The model under review builds one solid part; all positions refer to its coordinate system, in mm. Round coordinates to 2 decimals unless told otherwise and drop trailing zeros. Write each loop counter-clockwise with the first axis right and the second up, starting at its lowest first coordinate (ties: lowest second). Pieces come first, ordered by that corner, then holes. Notation, with made-up numbers: (56.25, 78) - (92.25, 78) arc R24 cw to (92.25, 96) - close; hole circle Ø4 at (-30.5, 8). An arc over 180 degrees is marked (long way). Return JSON: item names as keys, results as strings.
from build123d import *

# Parameters (mm, degrees)
F0_W     = 812.8
F0_H     = 304.8
F0_R     = 2.6924
F0_R_2   = 45.7835
F1_DEPTH = 3.81


with BuildPart() as f1:
    # F0 (on Top) → F1 (new body)
    with BuildSketch(Plane.XY):
        with Locations((314.836944, 203.638772)):
            Rectangle(F0_W, F0_H)
        with Locations((543.436944, 190.938772)):
            Circle(F0_R, mode=Mode.SUBTRACT)
        with Locations((619.636944, 190.938772)):
            Circle(F0_R, mode=Mode.SUBTRACT)
        with Locations((10.036944, 267.138772)):
            Circle(F0_R_2, mode=Mode.SUBTRACT)
        with Locations((543.436944, 305.238772)):
            Circle(F0_R, mode=Mode.SUBTRACT)
        with Locations((619.636944, 305.238772)):
            Circle(F0_R, mode=Mode.SUBTRACT)
    extrude(amount=F1_DEPTH)


solid = f1.part
(1) Add section A-A (y = 245.5). Write out the cut boundary in (x, z), plus the area to 3 significant figures.
Filled in:
{"outline": "(-91.56, 0) - (-30.31, 0) - (-30.31, 3.81) - (-91.56, 3.81) - close; (50.38, 0) - (721.24, 0) - (721.24, 3.81) - (50.38, 3.81) - close", "area": "2,790 mm2"}
(2) Clearance check with flat-ended pins moving along their axes: pin 1 Ø6 at (x, y) = (619.64, 305.24) entering from -Z; pin 2 Ø4.5 at (x, y) = (543.44, 190.94) entering from +Z. State where each tip first meets the part, or that it passes through.
Filled in:
{"pin 1": "stops at z = 0", "pin 2": "passes through"}
(3) Add section C-C (y = 295). Write out the cut boundary in (x, z), plus the area to 3 significant figures.
Filled in:
{"outline": "(-91.56, 0) - (-26.29, 0) - (-26.29, 3.81) - (-91.56, 3.81) - close; (46.37, 0) - (721.24, 0) - (721.24, 3.81) - (46.37, 3.81) - close", "area": "2,820 mm2"}
(4) Mouldability with a two-part tool opening along Y and no side actions: class faces 1 (the cylindrical face through (0.112, 222.444, 1.878)), 2 (the flat face through (309, 206, 3.81)) as released by +Y, released by -Y, zero draft, split by the parting line, or undercut.
Filled in:
{"face 1": "undercut", "face 2": "zero draft"}
(5) Wall thickness on line 1 (X direction, y = 307, z = 2.1); line 2 (Y direction, x = 33, z = 3.05); line 3 (X direction, y = 253, z = 3.6): over which ranges is each line inside the solid? List them lowest first.
Filled in:
{"line 1": "x = -91.56 to -12.48, 32.56 to 541.4, 545.47 to 617.6, 621.67 to 721.24", "line 2": "y = 51.24 to 227.53, 306.75 to 356.04", "line 3": "x = -91.56 to -33.51, 53.58 to 721.24"}
(6) Add section B-B (z = 2.9). Write out the cut boundary in (x, y), plus the area to 3 significant figures.
Filled in:
{"outline": "(-91.56, 51.24) - (721.24, 51.24) - (721.24, 356.04) - (-91.56, 356.04) - close; hole circle Ø91.57 at (10.04, 267.14); hole circle Ø5.38 at (543.44, 190.94); hole circle Ø5.38 at (543.44, 305.24); hole circle Ø5.38 at (619.64, 190.94); hole circle Ø5.38 at (619.64, 305.24)", "area": "241,000 mm2"}
